```python
from build123d import *

# Parameters (mm, degrees)
SKETCH1_W           = 106.5
SKETCH1_H           = 266
BOSS_EXTRUDE1_DEPTH = 2
SKETCH2_R           = 10
CUT_EXTRUDE1_DEPTH  = 10
SKETCH5_R           = 17.221351736
BOSS_EXTRUDE3_DEPTH = 0.75
FILLET2_R           = 0.5
CUT_EXTRUDE3_START  = -0.75
SKETCH6_R           = 10
CUT_EXTRUDE3_DEPTH  = 0.75


with BuildPart() as part:
    # Sketch1 → Boss-Extrude1 (new body)
    with BuildSketch(Plane.XY):
        with Locations((53.25, -133)):
            Rectangle(SKETCH1_W, SKETCH1_H)
    extrude(amount=BOSS_EXTRUDE1_DEPTH)

    # Sketch2 → Cut-Extrude1 (cut)
    with BuildSketch(Plane.XY.offset(2)):
        with Locations((81.5, -141)):
            Circle(SKETCH2_R)
    extrude(amount=-CUT_EXTRUDE1_DEPTH, mode=Mode.SUBTRACT)

    # Sketch5 → Boss-Extrude3 (add)
    with BuildSketch(Plane.XY.offset(2)):
        with Locations((81.5, -141)):
            Circle(SKETCH5_R)
    extrude(amount=BOSS_EXTRUDE3_DEPTH)

    # Fillet2
    fillet2_edges = [part.edges().sort_by_distance(p)[0] for p in [
        (64.278648264, -141, 2),
    ]]
    fillet(fillet2_edges, radius=FILLET2_R)

    # Sketch6 → Cut-Extrude3 (cut)
    with BuildSketch(Plane(origin=(0, 0, 2), x_dir=(-1, 0, 0), z_dir=(0, 0, -1)).offset(CUT_EXTRUDE3_START)):
        with Locations(Location((-81.5, -141, 0), (0, 0, 180))):
            Circle(SKETCH6_R)
    extrude(amount=CUT_EXTRUDE3_DEPTH, mode=Mode.SUBTRACT)


solid = part.part
```
The listing builds one solid part. Answer for the finished solid, in the listing's coordinates (mm). Coordinates: 2 decimals unless noted, no trailing zeros. Write each loop counter-clockwise with the first axis right and the second up, starting at its lowest first coordinate (ties: lowest second). Pieces come first, ordered by that corner, then holes.
Q1. Find the intervals of material crossed by line 1 along Y through (x, z) = (81.5, 0.75); line 2 along Y through (x, z) = (81.5, 2.35); line 3 along Z through (x, y) = (12, -127), in increasing order.
Returned:
line 1: y = -266 to -151, -131 to 0
line 2: y = -158.24 to -151, -131 to -123.76
line 3: z = 0 to 2
Q2. Given P1, Ø2, axis at x = 64, y = -32, coming from the -Z side, flat-ended and moving along its own axis, determine where the tip first touches the part or whether it passes through.
Returned:
P1: stops at z = 0
Q3. Section B-B, the plane x = 81.5 is taken. Write down the section's boundary in (y, z), then the cut area to 3 significant figures.
Returned:
outline: (-266, 0) - (-151, 0) - (-151, 2.75) - (-158.22, 2.75) - (-158.22, 2.5) arc R0.5 cw to (-158.72, 2) - (-266, 2) - close; (-131, 0) - (0, 0) - (0, 2) - (-123.28, 2) arc R0.5 cw to (-123.78, 2.5) - (-123.78, 2.75) - (-131, 2.75) - close
area: 503 mm2
Q4. Section D-D, the plane x = 18.5 is taken. Write down the section's boundary in (y, z).
Returned:
outline: (-266, 0) - (0, 0) - (0, 2) - (-266, 2) - close
Q5. Section A-A, the plane y = -141 is taken. Write down the section's boundary in (x, z), then the cut area to 3 significant figures.
Returned:
outline: (0, 0) - (71.5, 0) - (71.5, 2.75) - (64.28, 2.75) - (64.28, 2.5) arc R0.5 cw to (63.78, 2) - (0, 2) - close; (91.5, 0) - (106.5, 0) - (106.5, 2) - (99.22, 2) arc R0.5 cw to (98.72, 2.5) - (98.72, 2.75) - (91.5, 2.75) - close
area: 184 mm2
Q6. Section C-C, the plane y = -86 is taken. Write down the section's boundary in (x, z).
Returned:
outline: (0, 0) - (106.5, 0) - (106.5, 2) - (0, 2) - close
